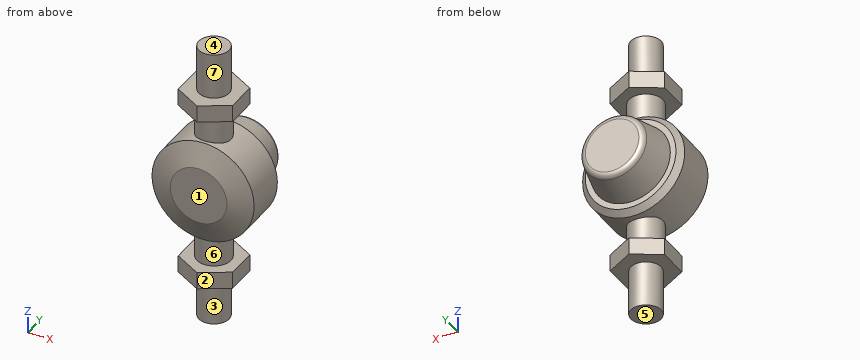
```python
from build123d import *

# Parameters (mm, degrees)
EXTRUDE_324_DEPTH = 15
SKETCH_2_R        = 15
EXTRUDE_1_DEPTH   = 140
EXTRUDE_2_DEPTH   = 15
SKETCH_4_R        = 13.4
EXTRUDE_3_DEPTH   = 40
EXTRUDE_START     = 40
SKETCH_5_R        = 13.4
EXTRUDE_4_DEPTH   = 40
SKETCH_6_R        = 45
EXTRUDE_5_DEPTH   = 25
CHAMFER_1_SIZE    = 20
CHAMFER_1_SIZE2   = 7.279404685
CHAMFER_2_SIZE    = 5
SKETCH_7_R        = 27.5
SKETCH_8_R        = 35
FILLET_1_R        = 5


with BuildPart() as part:
    # Эскиз1 → Extrude 324 (new body)
    with BuildSketch(Plane.XY):
        Polygon((0, 27.712812921), (-24, 13.856406461), (-24, -13.856406461), (0, -27.712812921), (24, -13.856406461), (24, 13.856406461), align=None)
    extrude(amount=-EXTRUDE_324_DEPTH)

    # Эскиз2 → Бобышка-Вытянуть1 (add)
    with BuildSketch(Plane(origin=(0, 0, -15), x_dir=(-1, 0, 0), z_dir=(0, 0, -1))):
        Circle(SKETCH_2_R)
    extrude(amount=EXTRUDE_1_DEPTH)

    # Эскиз3 → Бобышка-Вытянуть2 (add)
    with BuildSketch(Plane(origin=(0, 0, -155), x_dir=(-1, 0, 0), z_dir=(0, 0, -1))):
        Polygon((0, 27.712812921), (-24, 13.856406461), (-24, -13.856406461), (0, -27.712812921), (24, -13.856406461), (24, 13.856406461), align=None)
    extrude(amount=EXTRUDE_2_DEPTH)

    # Эскиз4 → Бобышка-Вытянуть3 (add)
    with BuildSketch(Plane.XY):
        with Locations(Location((0, 0, 0), (0, 0, 180))):
            Circle(SKETCH_4_R)
    extrude(amount=EXTRUDE_3_DEPTH)

    # Эскиз5 → Бобышка-Вытянуть4 (add)
    with BuildSketch(Plane(origin=(0, 0, -170), x_dir=(-1, 0, 0), z_dir=(0, 0, -1)).offset(EXTRUDE_START)):
        Circle(SKETCH_5_R)
    extrude(amount=-EXTRUDE_4_DEPTH)

    # Эскиз6 → Бобышка-Вытянуть5 (add, symmetric)
    with BuildSketch(Plane(origin=(0, 0, 0), x_dir=(1, 0, 0), z_dir=(0, 1, 0))):
        with Locations(Location((0, 85, 0), (0, 0, 270))):
            Circle(SKETCH_6_R)
    extrude(amount=EXTRUDE_5_DEPTH, both=True)

    # Фаска1
    chamfer_1_edges = [part.edges().sort_by_distance(p)[0] for p in [
        (0, -25, -130),
    ]]
    chamfer_1_side = [part.faces().sort_by_distance(p)[0] for p in [
        (0, -25, -85),
    ]]
    chamfer(chamfer_1_edges, length=CHAMFER_1_SIZE, length2=CHAMFER_1_SIZE2, reference=chamfer_1_side[0])

    # Фаска2
    chamfer_2_edges = [part.edges().sort_by_distance(p)[0] for p in [
        (0, 25, -130),
    ]]
    chamfer(chamfer_2_edges, length=CHAMFER_2_SIZE)

    # Эскиз7 → Бобышка-По сечениям1 section 0
    with BuildSketch(Plane(origin=(0, 55, 0), x_dir=(-1, 0, 0), z_dir=(0, 1, 0))):
        with Locations((0, -85)):
            Circle(SKETCH_7_R)
    # Эскиз8 → Бобышка-По сечениям1 section 1
    with BuildSketch(Plane(origin=(0, 25, 0), x_dir=(-1, 0, 0), z_dir=(0, 1, 0))):
        with Locations((0, -85)):
            Circle(SKETCH_8_R)
    loft()

    # Скругление1
    fillet_1_edges = [part.edges().sort_by_distance(p)[0] for p in [
        (27.5, 55, -85),
    ]]
    fillet(fillet_1_edges, radius=FILLET_1_R)


solid = part.part
```
Could you check a few things on this model? Use its own coordinates, in mm. Face numbers are marked on the shaded views. A direction names the side the tool comes from. Coordinates: 2 decimals unless noted, no trailing zeros. Order: outer loops, then holes, each group sorted by start corner. A loop starts at its lowest first (then second) coordinate and runs counter-clockwise, first axis right, second up. Notation, with made-up numbers: M 34,62.25 L 47,62.25 A19 cw 47,98.25 Z; hole C -10,21.25 d2. An arc over 180 degrees is marked long. Use a Markdown table: item, result. Add a question column.
Q1. I'm going to push flat-ended pins straight in: pin 1 (8 mm diameter, centred on x = 9.5, y = 30, fed in from -Z); pin 2 (7.5 mm diameter, centred on y = 0, z = -164, fed in from -X); pin 3 (6 mm diameter, centred on x = -16, y = 6, fed in from +Z). Where does each tip first touch, or does it pass through?
Q2. Which directions (+Z, -Z, +X, -X, +Y, -Y) give clear straight access to the entire face, cutting with the end or side of a thin tool? Please do the marked faces 1, 2 and 3.
Q3. I want a section at B-B on z = -5. List the corners of the cut face in (x, y) for me, then the cut area to 3 significant figures.
Q4. I want a section at A-A on y = 0. List the corners of the cut face in (x, z) for me, then the cut area to 3 significant figures.
Q5. If I drill on L1, parallel to Z at x = -2, y = 16.5; L2, parallel to Z at x = 19.5, y = -14; L3, parallel to X at y = 0.5, z = 4, over which ranges is the centre line in solid material (lowest first)?
Q6. I want a section at C-C on z = -193.5. List the corners of the cut face in (x, y) for me, then the cut area to 3 significant figures.
Q7. We'd pull the mould along Z, two halves only. Please class the marked faces 4, 5, 6 and 7: pulls with the +Z half, pulls with the -Z half, needs draft (parallel to the pull), parting line crosses it, or undercut.
Q8. I want a section at D-D on z = -152. List the corners of the cut face in (x, y) for me, then the cut area to 3 significant figures.
Checked values:
| question | item | result |
|---|---|---|
| 1 | pin 1 | z = -118.81 |
| 1 | pin 2 | x = -24 |
| 1 | pin 3 | z = 0 |
| 2 | face 1 | +X, -X, -Y |
| 2 | face 2 | -Z, +X, -Y |
| 2 | face 3 | -Z |
| 3 | outline | M -24,-13.86 L 0,-27.71 L 24,-13.86 L 24,13.86 L 0,27.71 L -24,13.86 Z |
| 3 | area | 2,000 mm² |
| 4 | outline | M -24,-170 L -13.4,-170 L -13.4,-210 L 13.4,-210 L 13.4,-170 L 24,-170 L 24,-155 L 15,-155 L 15,-127.43 A45 ccw 15,-42.57 L 15,-15 L 24,-15 L 24,0 L 13.4,0 L 13.4,40 L -13.4,40 L -13.4,0 L -24,0 L -24,-15 L -15,-15 L -15,-42.57 A45 ccw -15,-127.43 L -15,-155 L -24,-155 Z |
| 4 | area | 11,500 mm² |
| 5 | L1 | -170 to -155, -129.96 to -40.04, -15 to 0 |
| 5 | L2 | -170 to -155, -125.56 to -44.44, -15 to 0 |
| 5 | L3 | -13.39 to 13.39 |
| 6 | outline | C 0,0 d26.8 |
| 6 | area | 564 mm² |
| 7 | face 4 | pulls with the +Z half |
| 7 | face 5 | pulls with the -Z half |
| 7 | face 6 | undercut |
| 7 | face 7 | needs draft |
| 8 | outline | C 0,0 d30 |
| 8 | area | 707 mm² |
